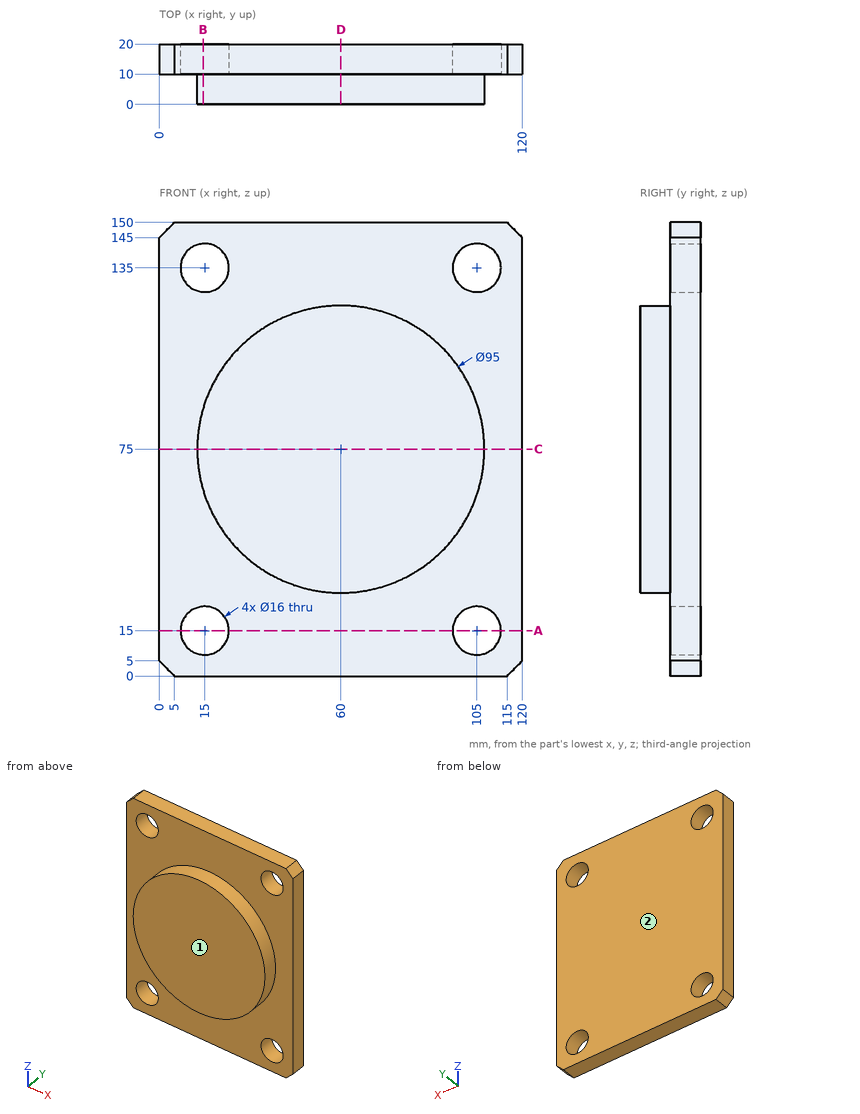
Part print with two shaded views. Sizes in mm from the minimum x, y, z corner. Coordinates: 2 decimals unless noted, no trailing zeros. Order: outer loops, then holes, each group sorted by start corner. A loop starts at its lowest first (then second) coordinate and runs counter-clockwise, first axis right, second up. Notation, with made-up numbers: (66.25, -6.5) - (112.25, -6.5) arc R26 ccw to (112.25, 26.5) - close; hole circle Ø7 at (38.5, 36). An arc over 180 degrees is marked (long way). Answer in a Markdown table with one row per item.
1. Slice it at B-B, the plane x = 14.5. List the corners of the cut face in (y, z).
Answer:
| item | result |
|---|---|
| outline | (0, 61.36) - (10, 61.36) - (10, 22.98) - (20, 22.98) - (20, 127.02) - (10, 127.02) - (10, 88.64) - (0, 88.64) - close; (10, 0) - (20, 0) - (20, 7.02) - (10, 7.02) - close; (10, 142.98) - (20, 142.98) - (20, 150) - (10, 150) - close |
2. Drill centre lines: L1, parallel to Z at x = 15, y = 14.5; L2, parallel to Y at x = 111, z = 42; L3, parallel to X at y = 12.5, z = 22. Where is each one in solid material? Low to high. Write a range as from..to.
Answer:
| item | result |
|---|---|
| L1 | 0..7, 23..127, 143..150 |
| L2 | 10..20 |
| L3 | 0..11.13, 18.87..101.13, 108.87..120 |
3. Slice it at A-A, the plane z = 15. List the corners of the cut face in (x, y), then the cut area to 3 significant figures.
Answer:
| item | result |
|---|---|
| outline | (0, 10) - (7, 10) - (7, 20) - (0, 20) - close; (23, 10) - (97, 10) - (97, 20) - (23, 20) - close; (113, 10) - (120, 10) - (120, 20) - (113, 20) - close |
| area | 880 mm² |
4. Slice it at D-D, the plane x = 60. List the corners of the cut face in (y, z), then the cut area to 3 significant figures.
Answer:
| item | result |
|---|---|
| outline | (0, 27.5) - (10, 27.5) - (10, 0) - (20, 0) - (20, 150) - (10, 150) - (10, 122.5) - (0, 122.5) - close |
| area | 2,450 mm² |
5. Slice it at C-C, the plane z = 75. List the corners of the cut face in (x, y), then the cut area to 3 significant figures.
Answer:
| item | result |
|---|---|
| outline | (0, 10) - (12.5, 10) - (12.5, 0) - (107.5, 0) - (107.5, 10) - (120, 10) - (120, 20) - (0, 20) - close |
| area | 2,150 mm² |
6. Pull direction Y, two halves, no side cores. Call the marked faces 1 and 2: +Y half, -Y half, draft (parallel to the pull), parting line (faces both ways), or undercut.
Answer:
| item | result |
|---|---|
| face 1 | -Y half |
| face 2 | +Y half |
7. Flat gauge pins, fed straight in: P1, Ø12, axis at y = 2.5, z = 134.5, coming from the +X side; P2, Ø21, axis at x = 105, z = 15, coming from the -Y side; P3, Ø1, axis at y = 3, z = 59.5, coming from the +X side; P4, Ø8, axis at x = 23.5, y = 2, coming from the -Z side. Where does each tip first touch, or does it go through?
Answer:
| item | result |
|---|---|
| P1 | through |
| P2 | y = 10 |
| P3 | x = 105.07 |
| P4 | z = 40.36 |
